Autodesk Inventor part; units mm, degrees
ref_plane "YZ Plane" through (0, 0, 0) normal (1, 0, 0) x (0, 1, 0)
ref_plane "XZ Plane" through (0, 0, 0) normal (0, 1, 0) x (-1, 0, 0)
ref_plane "XY Plane" through (0, 0, 0) normal (0, 0, 1) x (1, 0, 0)
sketch "Sketch1" plane through (0, 0, 0) normal (0, 1, 0) x (-1, 0, 0)
  line L0 (62, 0) -> (-57, 0)
  line L1 (0, -63) -> (0, 63)
  line L2 (9.25, 17.5) -> (-9.25, 17.5)
  line L3 (-9.25, 17.5) -> (-9.25, -17.5)
  line L4 (-9.25, -17.5) -> (9.25, -17.5)
  line L5 (9.25, -17.5) -> (9.25, 17.5)
  circle A0 centre (0, 0) radius 33.5
  circle A1 centre (0, 0) radius 27
  line L6 (0, 45) -> (-40, 45)
  line L7 (-40, 45) -> (-40, -45)
  line L8 (-40, -45) -> (0, -45)
  arc A2 (0, -45) -> (0, 45) centre (0, 0) ccw
  line L9 (-13.1237, -34.8874) -> (-27, -34.8874)
  line L10 (-27, -34.8874) -> (-27, -24.7237)
  line L11 (-27, -24.7237) -> (-22.6051, -24.7237)
  line L12 (-13.1237, -30.8224) -> (-13.1237, -34.8874)
  circle A3 centre (-27.7874, 31.6695) radius 3.05
  circle A4 centre (-27.7874, 31.6695) radius 5
  line L13 (0, 40) -> (-35, 40)
  line L14 (-35, -40) -> (0, -40)
  arc A5 (0, -40) -> (0, 40) centre (0, 0) ccw
  line L15 (-35, -38) -> (0, -38)
  arc A6 (0, -38) -> (0, 38) centre (0, 0) ccw
  line L16 (0, 38) -> (-35, 38)
  line L17 (-35, -40) -> (-35, -38)
  line L18 (-35, 38) -> (-35, 40)
  dimension "d0" = 18.5
  dimension "d1" = 35
  dimension "d2" = 67
  dimension "d3" = 54
  dimension "d18" = 6.1
  dimension "d19" = 10
  dimension "d26" = 2
extrude "Extrusion1" add sketch "Sketch1" along normal blind 5 contours A0 L1 A6 L0 | L0 A6 L1 A0 | A1 L1 L4 L5 L0 | L0 L5 L2 L1 A1 | A6 L1 A5 L0 | L0 A5 L1 A6 | A0 L0 L7 L6 L1 L13 L18 L16 | L1 L15 L17 L14 L8 L7 L0 A0 L11 L10 L9 L12 | L1 L2 L3 L0 A1 | A1 L0 L3 L4 L1 | A5 L1 A2 L0 | L0 A2 L1 A5 | L1 L14 L17 L15 | L16 L18 L13 L1 | L12 L9 L10 L11 A0 | A3 | A4
sketch "Sketch2" plane through (0, 5, 0) normal (0, 1, 0) x (1, 0, 0)
  line L0 (40, 45) -> (0, 45)
  arc A0 (0, 45) -> (0, -45) centre (0, 0) ccw
  line L1 (0, -45) -> (40, -45)
  line L2 (40, -45) -> (40, 45)
extrude "Extrusion2" add sketch "Sketch2" along normal blind 1
sketch "Sketch3" plane through (0, 5, 0) normal (0, -1, 0) x (1, 0, 0)
  line L0 (-9.25, -17.5) -> (9.25, -17.5)
  line L1 (9.25, -17.5) -> (9.25, 17.5)
  line L2 (9.25, 17.5) -> (-9.25, 17.5)
  line L3 (-9.25, 17.5) -> (-9.25, -17.5)
  point P0 (0, 0)
extrude "Extrusion3" cut sketch "Sketch3" against normal through all
extrude "Extrusion4" cut sketch "Sketch1" along normal blind 5 contours L12 L9 L10 L11 A0
sketch "Sketch4" plane through (0, 0, 0) normal (0, -1, 0) x (1, 0, 0)
  line L0 (40, -45) -> (0, -45)
  line L1 (40, 45) -> (40, -45)
  line L2 (0, 45) -> (40, 45)
  line L3 (40, -45) -> (37, -45)
  line L4 (37, -45) -> (37, 45)
  line L5 (37, 45) -> (40, 45)
  line L6 (40, 45) -> (40, -45)
  dimension "d14" = 3
extrude "Extrusion5" add sketch "Sketch4" along normal blind 80
extrude "Extrusion6" add sketch "Sketch1" against normal blind 8 contours A4
extrude "Extrusion8" add sketch "Sketch1" against normal blind 20 contours A6 L1 A5 L0 | L0 A5 L1 A6 | L1 L14 L17 L15 | L16 L18 L13 L1
sketch "Sketch5" plane through (37, 0, -45) normal (-1, 0, 0) x (0, 0, 1)
  line L0 (0, -80) -> (90, -80)
  line L1 (37.5, -80) -> (52.5, -80)
  line L2 (52.5, -80) -> (52.5, -74)
  line L3 (52.5, -74) -> (37.5, -74)
  line L4 (37.5, -74) -> (37.5, -80)
  line L5 (0, 0) -> (0, -80)
  circle A0 centre (25.7628, -15.894) radius 1
  circle A1 centre (25.7628, -15.894) radius 2.5
  line L6 (25.7628, -7.1865) -> (25.7628, -27.0145) construction
  line L7 (25.7628, -15.894) -> (50.5115, -40.6428) construction
  line L8 (25.7628, -15.894) -> (60.7628, -15.894) construction
  circle A2 centre (50.5115, -40.6428) radius 1 construction
  circle A3 centre (50.5115, -40.6428) radius 2.5 construction
  circle A4 centre (50.5115, -40.6428) radius 1
  circle A5 centre (50.5115, -40.6428) radius 2.5
  dimension "d29" = 15
  dimension "d30" = 6
  dimension "d31" = 37.5
  dimension "d37" = 2
  dimension "d38" = 5
  dimension "d39" = 35
  dimension "d40" = 45
  dimension "d41" = 2
  dimension "d42" = 5
extrude "Extrusion9" add sketch "Sketch5" along normal blind 20 contours L4 L3 L2 L0
sketch "Sketch6" plane through (0, -80, 0) normal (0, -1, 0) x (1, 0, 0)
  circle A0 centre (27, 0) radius 1
  point P0 (0, 0)
  dimension "d34" = 2
extrude "Extrusion10" cut sketch "Sketch6" against normal blind 5
extrude "Extrusion11" add sketch "Sketch5" along normal blind 5 contours A1 | A5
properties part number "Celo_3DPrint"
The model under review builds one solid part; all positions refer to its coordinate system, in mm. A direction names the side the tool comes from. Round coordinates to 2 decimals unless told otherwise and drop trailing zeros. Loops run counter-clockwise (first coordinate to the right, second up) from the corner with the lowest first, then second, coordinate; pieces in that order, holes last. Notation, with made-up numbers: M 50,43 L 102,43 A29 cw 102,65 Z; hole C 18.25,74.5 d5. An arc over 180 degrees is marked long. Answer as a JSON object with one key per item and string values.
Item 1: We need section A-A, the plane y = -1.5. State the section outline as (x, z) points, and give its area (3 significant figures).
Check sheet entries:
{"outline": "M 0,-40 L 35,-40 L 35,-38 L 0,-38 A38 cw 0,38 L 35,38 L 35,40 L 0,40 A40 ccw Z; C 27.79,31.67 d10; M 37,-45 L 40,-45 L 40,45 L 37,45 Z; hole C 27.79,31.67 d6.1", "area": "704 mm2"}
Item 2: Clearance check with flat-ended pins moving along their axes: P1, Ø4, axis at y = -15, z = -18, coming from the -X side; P2, Ø10, axis at x = 26, y = -14.5, coming from the -Z side; P3, Ø1.6, axis at y = -40.64, z = 5.51, coming from the -X side; P4, Ø1, axis at x = 27.5, z = 0.5, coming from the -Y side. State where each tip first meets the part, or that it passes through.
Check sheet entries:
{"P1": "x = -36.66", "P2": "z = -40", "P3": "x = 37", "P4": "y = -80"}
Item 3: We need section D-D, the plane z = 24. State the section outline as (x, y) points, and give its area (3 significant figures).
Check sheet entries:
{"outline": "M -38.07,0 L -32,0 L -32,-20 L -29.46,-20 L -29.46,0 L -23.37,0 L -23.37,5 L -12.37,5 L -12.37,0 L 12.37,0 L 12.37,5 L 23.37,5 L 23.37,0 L 37,0 L 37,-80 L 40,-80 L 40,6 L -38.07,6 Z", "area": "649 mm2"}
Item 4: The part is to be moulded in two halves that separate along Z. For faces 5 (the face through (17, -10, 40)), 6 (the face through (18, -10, -38)), 7 (the face through (-13, 6, -1)), say which applies: +Z half, -Z half, draft (parallel to the pull), parting line (faces both ways), or undercut.
Check sheet entries:
{"face 5": "+Z half", "face 6": "undercut", "face 7": "draft"}
Item 5: For line 1 along Z through (x, y) = (27, -78); line 2 along X through (y, z) = (-71.5, 36); line 3 along Y through (x, z) = (31.5, -28), list the stretches that pass through material, from the lowest coordinate up.
Check sheet entries:
{"line 1": "-7.5 to -1, 1 to 7.5", "line 2": "37 to 40", "line 3": "0 to 6"}
Item 6: Tool access review of faces 1 (the face through (-9.25, 3, 0)), 2 (the face through (-38.4, -20, 0.2)), 3 (the face through (20, 2, -34.887)), 4 (the face through (27, -77, 7.5)): name each direction out of +Z, -Z, +X, -X, +Y, -Y from which nothing blocks a thin tool from reaching the whole face with its end or side.
Check sheet entries:
{"face 1": "+Y, -Y", "face 2": "+Z, -Z, -X, -Y", "face 3": "-Y", "face 4": "+Z, -X, -Y"}
Item 7: We need section B-B, the plane x = 18.5. State the section outline as (y, z) points.
Check sheet entries:
{"outline": "M -80,-7.5 L -74,-7.5 L -74,7.5 L -80,7.5 Z; M -20,-40 L 0,-40 L 0,-45 L 6,-45 L 6,45 L 0,45 L 0,40 L -20,40 L -20,38 L 0,38 L 0,27.93 L 5,27.93 L 5,19.67 L 0,19.67 L 0,-19.67 L 5,-19.67 L 5,-34.89 L 0,-34.89 L 0,-38 L -20,-38 Z"}
Item 8: We need section C-C, the plane x = -30. State the section outline as (y, z) points.
Check sheet entries:
{"outline": "M -20,-26.46 L 0,-26.46 L 0,-33.54 L 6,-33.54 L 6,33.54 L 0,33.54 L 0,26.46 L -20,26.46 L -20,23.32 L 0,23.32 L 0,14.91 L 5,14.91 L 5,-14.91 L 0,-14.91 L 0,-23.32 L -20,-23.32 Z"}
